Can you work these out from the model? Positions are in its coordinate system, mm. A direction names the side the tool comes from. Coordinates: 2 decimals unless noted, no trailing zeros. Order: outer loops, then holes, each group sorted by start corner. A loop starts at its lowest first (then second) coordinate and runs counter-clockwise, first axis right, second up. Notation, with made-up numbers: (-26.75, 56.25) -> (20.25, 56.25) arc R11 cw to (20.25, 73.25) -> close; hole circle Ø1 at (27.5, -25). An arc over 180 degrees is marked (long way). Use a Markdown table: item, result. Add a question column.
1. Suppose I cut it at A-A, the plane y = 18. List the corners of the cut face in (x, z) for me.
2. We'd pull the mould along X, two halves only. Please class faces 6 (the flat face through (23, -24.35, 30)), 7 (the flat face through (15, -6, 37)), 8 (the cylindrical face through (106.996, 12.254, 7.395)): pulls with the +X half, pulls with the -X half, needs draft (parallel to the pull), parting line crosses it, or undercut.
3. If I drill on line 1 along X through (y, z) = (14.5, 58); line 2 along Y through (x, z) = (-89, 11.75); line 3 along Z through (x, y) = (-78, -1), over which ranges is the centre line in solid material (lowest first)? Write a range as from..to.
4. Suppose I cut it at C-C, the plane x = 9.5. List the corners of the cut face in (y, z) for me.
5. Suppose I cut it at B-B, the plane z = 9.5. List the corners of the cut face in (x, y) for me, then the cut area to 3 significant figures.
6. For pin 1 Ø2 at (y, z) = (16.5, 49) entering from -X; pin 2 Ø10 at (y, z) = (-11.5, 13) entering from +X; pin 3 Ø7.5 at (x, z) = (49, 5.5) entering from -Y; pin 4 Ø23.5 at (x, y) = (-89, 12.65) entering from -Z, each with a flat end and sliding along its axis, tell me the tip position at first contact or that it passes through.
7. For faces 1 (the flat face through (68, 13, 15)), 2 (the flat face through (59, -5.35, 7)), 3 (the flat face through (-15, -6, 37)), 4 (the flat face through (-60, -5.35, 7)), 5 (the flat face through (-61, 13, 15)), which set-ups out of +Z, -Z, +X, -X, +Y, -Y let a thin tool reach every point of the face, with its end or its side?
8. Suppose I cut it at D-D, the plane z = 25. List the corners of the cut face in (x, y) for me.
```python
from build123d import *

# Parameters (mm, degrees)
F1_DEPTH = 61
F0_R     = 9
F2_DEPTH = 15
F4_DEPTH = 30


with BuildPart() as f1:
    # F0 (on Top) → F1 (new body)
    with BuildSketch(Plane.XY):
        Polygon((30.5, 30.649616), (-30.5, 30.649616), (-30.5, -5.350384), (-30.5, -24.350384), (-15, -24.350384), (-15, -16.350384), (-15, 22.899616), (0, 22.899616), (15, 22.899616), (15, -16.350384), (15, -24.350384), (30.5, -24.350384), (30.5, -5.350384), align=None)
    extrude(amount=F1_DEPTH)

    # F0 (on Top) → F2 (join)
    with BuildSketch(Plane.XY):
        with BuildLine():
            Line((89, 30.649616), (30.5, 30.649616))
            Line((30.5, 30.649616), (30.5, -5.350384))
            Line((30.5, -5.350384), (89, -5.350384))
            ThreePointArc((89, -5.350384), (107, 12.649616), (89, 30.649616))
        make_face()
        with Locations((89, 12.649616)):
            Circle(F0_R, mode=Mode.SUBTRACT)
        with BuildLine():
            Line((-30.5, -5.350384), (-30.5, 30.649616))
            Line((-30.5, 30.649616), (-89, 30.649616))
            ThreePointArc((-89, 30.649616), (-107, 12.649616), (-89, -5.350384))
            Line((-89, -5.350384), (-30.5, -5.350384))
        make_face()
        with Locations((-89, 12.649616)):
            Circle(F0_R, mode=Mode.SUBTRACT)
    extrude(amount=F2_DEPTH)

    # F3 (on face) → F4 (join)
    with BuildSketch(Plane.YZ.offset(-15)):
        Polygon((22.899616, 0), (22.899616, 61), (-16.350384, 0), align=None)
    extrude(amount=F4_DEPTH)


solid = f1.part
```
Worked out:
| question | item | result |
|---|---|---|
| 1 | outline | (-106.19, 0) -> (-96.24, 0) -> (-96.24, 15) -> (-106.19, 15) -> close; (-81.76, 0) -> (81.76, 0) -> (81.76, 15) -> (30.5, 15) -> (30.5, 61) -> (15, 61) -> (15, 53.39) -> (-15, 53.39) -> (-15, 61) -> (-30.5, 61) -> (-30.5, 15) -> (-81.76, 15) -> close; (96.24, 0) -> (106.19, 0) -> (106.19, 15) -> (96.24, 15) -> close |
| 2 | face 6 | needs draft |
| 2 | face 7 | undercut |
| 2 | face 8 | pulls with the +X half |
| 3 | line 1 | x = -30.5..-15, 15..30.5 |
| 3 | line 2 | y = -5.35..3.65, 21.65..30.65 |
| 3 | line 3 | z = 0..15 |
| 4 | outline | (-16.35, 0) -> (30.65, 0) -> (30.65, 61) -> (22.9, 61) -> close |
| 5 | outline | (-89, -5.35) -> (-30.5, -5.35) -> (-30.5, -24.35) -> (-15, -24.35) -> (-15, -10.24) -> (15, -10.24) -> (15, -24.35) -> (30.5, -24.35) -> (30.5, -5.35) -> (89, -5.35) arc R18 ccw to (89, 30.65) -> (-89, 30.65) arc R18 ccw to start; hole circle Ø18 at (-89, 12.65); hole circle Ø18 at (89, 12.65) |
| 5 | area | 7,650 mm² |
| 6 | pin 1 | stops at x = -30.5 |
| 6 | pin 2 | stops at x = 30.5 |
| 6 | pin 3 | stops at y = -5.35 |
| 6 | pin 4 | stops at z = 0 |
| 7 | face 1 | +Z, +X, +Y, -Y |
| 7 | face 2 | +Z, -Z, +X, -Y |
| 7 | face 3 | +Z, -Y |
| 7 | face 4 | +Z, -Z, -X, -Y |
| 7 | face 5 | +Z, -X, +Y, -Y |
| 8 | outline | (-30.5, -24.35) -> (-15, -24.35) -> (-15, -0.26) -> (15, -0.26) -> (15, -24.35) -> (30.5, -24.35) -> (30.5, 30.65) -> (-30.5, 30.65) -> close |
